```python
from build123d import *

# Parameters (mm, degrees)
F1_DEPTH  = 25.4
F2_R      = 3.175
F3_DEPTH  = 6.35
F4_R      = 3.81
F5_R      = 2.54
F6_DEPTH  = 8.89
F8_R      = 2.54
F11_R     = 6.35
F12_DEPTH = 25.4


with BuildPart() as f1:
    # F0 (on Front) → F1 (new body)
    with BuildSketch(Plane.XZ):
        with BuildLine():
            Line((0, 66.4387534539), (0, 41.0387534539))
            ThreePointArc((0, 41.0387534539), (37.4494820277, 88.5304728284), (50.8, 147.5193767269))
            ThreePointArc((50.8, 147.5193767269), (37.4494820277, 206.5082806255), (0, 254))
            Line((0, 254), (0, 228.6))
            ThreePointArc((0, 228.6), (25.9369896247, 147.5193767269), (0, 66.4387534539))
        make_face()
        with BuildLine():
            ThreePointArc((0, 25.4), (7.4394877579, 7.4394877579), (25.4, 0))
            ThreePointArc((25.4, 0), (43.3605122421, 7.4394877579), (50.8, 25.4))
            Line((50.8, 25.4), (50.8, 147.5193767269))
            ThreePointArc((50.8, 147.5193767269), (37.4494820277, 88.5304728284), (0, 41.0387534539))
            Line((0, 41.0387534539), (0, 25.4))
        make_face()
    extrude(amount=F1_DEPTH)

    # F2 (on face) → F3 (cut)
    with BuildSketch(Plane.XZ.offset(25.4)):
        with Locations((25.4, 25.4)):
            Circle(F2_R)
    extrude(amount=-F3_DEPTH, mode=Mode.SUBTRACT)

    # F4
    f4_edges = [f1.edges().sort_by_distance(p)[0] for p in [
        (0, -12.7, 254),
        (0, -12.7, 228.6),
        (0, 0, 241.3),
        (0, -25.4, 241.3),
        (0, -12.7, 66.438753),
        (0, -12.7, 25.4),
        (0, 0, 45.919377),
        (0, -25.4, 45.919377),
    ]]
    fillet(f4_edges, radius=F4_R)

    # F5 (on face) → F6 (join)
    with BuildSketch(Plane.XZ.offset(25.4)):
        with Locations((26.6260020435, 191.9900625944)):
            Circle(F5_R)
        with Locations((41.8660020435, 161.5079194307)):
            Circle(F5_R)
    extrude(amount=F6_DEPTH)

    # F10: sweep along a path in F9
    with BuildLine(Plane.XY.offset(161.507932)) as f10_path:
        Line((41.8660020435, -34.29), (41.8660020435, -40.0177))
        ThreePointArc((41.8660020435, -40.0177), (40.9397858176, -42.2537837741), (38.7037020435, -43.18))
        Line((38.7037020435, -43.18), (28.5437020435, -43.18))
    # F8 (on face) → F10 (sweep)
    with BuildSketch(Plane.XZ.offset(34.29)):
        with Locations((41.8660020435, 161.5079194307)):
            Circle(F8_R)
    sweep(path=f10_path.line)

    # F11 (on face) → F12 (cut)
    with BuildSketch(Plane.XZ.offset(19.05)):
        with Locations((25.4, 25.4)):
            Circle(F11_R)
    extrude(amount=-F12_DEPTH, mode=Mode.SUBTRACT)


solid = f1.part
```
Geometry: final body of the model. Coordinates: model frame, mm. A direction names the side the tool comes from. Round coordinates to 2 decimals unless told otherwise and drop trailing zeros. Order: outer loops, then holes, each group sorted by start corner. A loop starts at its lowest first (then second) coordinate and runs counter-clockwise, first axis right, second up. Notation, with made-up numbers: (69.25, 14) -> (79.25, 14) arc R18 ccw to (79.25, 43) -> close; hole circle Ø8 at (-22.75, 36.25). An arc over 180 degrees is marked (long way). Write each question's results on one line, items separated by ' | '.
Q1. Pull-direction query (X, two-part tool) for faces 1 (the face through (0, -13, 238)), 2 (the face through (22, -19.05, 24)), 3 (the face through (20.36, -9.66, 21.54)), 4 (the face through (27.798, -29.783, 189.737)); classes: released by +X, released by -X, zero draft, split by the parting line, or undercut.
Response values:
face 1: released by -X | face 2: undercut | face 3: undercut | face 4: split by the parting line
Q2. Pin query (flat end, axial travel): pin 1 Ø16.5 at (x, z) = (25.4, 25.4) entering from -Y; pin 2 Ø12 at (y, z) = (-17, 222.5) entering from -X; pin 3 Ø12 at (x, y) = (45.5, -25) entering from -Z. Return the tip coordinate at first contact, or that it passes through.
Response values:
pin 1: y = -25.4 | pin 2: x = 0.23 | pin 3: z = 4.78
Q3. Section query A-A (y = -10). Output: boundary loops of the cut face in (x, z), and give its area (3 significant figures).
Response values:
outline: (0, 25.4) arc R25.4 ccw to (50.8, 25.4) -> (50.8, 147.52) arc R137 ccw to (6.38, 248.5) arc R3.81 ccw to (0, 245.69) -> (0, 229.81) arc R3.81 ccw to (0.69, 227.63) arc R139.7 cw to (0.69, 67.41) arc R3.81 ccw to (0, 65.23) -> close; hole circle Ø12.7 at (25.4, 25.4) | area: 7,980 mm²
Q4. Access query for faces 5 (the face through (33.553, -44.545, 163.65)), 6 (the face through (50.8, -13, 86)), 7 (the face through (28.544, -43, 162)). Directions: +Z, -Z, +X, -X, +Y, -Y. A direction counts if a zero-diameter tool reaches every point of the face in a straight line with its end or side. Return the directions, or none.
Response values:
face 5: -X | face 6: +Z, -Z, +X, +Y, -Y | face 7: +Z, -Z, -X, -Y
Q5. Ray query, line 1 along X through (y, z) = (-20, 25); line 2 along X through (y, z) = (-13, 25); line 3 along Y through (x, z) = (21, 91). Return the intervals inside material, ascending.
Response values:
line 1: 0 to 22.25, 28.55 to 50.8 | line 2: 0 to 19.06, 31.74 to 50.8 | line 3: -25.4 to 0
